Input: part model. Units: mm. Frame: model coordinates. A direction names the side the tool comes from. Coordinates: 2 decimals unless noted, no trailing zeros. Loops run counter-clockwise (first coordinate to the right, second up) from the corner with the lowest first, then second, coordinate; pieces in that order, holes last.
```python
from build123d import *

# Parameters (mm, degrees)
SKETCH_1_R          = 8
SKETCH_1_R_2        = 3
EXTRUDE_1_DEPTH     = 11
SKETCH_2_W          = 1.4
SKETCH_2_H          = 7.329379883
CUT_EXTRUDE_1_DEPTH = 13.5
SKETCH_3_R          = 1
CUT_EXTRUDE_2_DEPTH = 3.5
SKETCH_4_R          = 1.6
EXTRUDE_3_DEPTH     = 2


with BuildPart() as part:
    # 草图1 → 凸台-拉伸1 (new body)
    with BuildSketch(Plane.XY):
        Circle(SKETCH_1_R)
        Circle(SKETCH_1_R_2, mode=Mode.SUBTRACT)
    extrude(amount=EXTRUDE_1_DEPTH)

    # 草图2 → 切除-拉伸1 (cut)
    with BuildSketch(Plane.XY.offset(11)):
        with Locations((0, 5.87801753)):
            Rectangle(SKETCH_2_W, SKETCH_2_H)
    extrude(amount=-CUT_EXTRUDE_1_DEPTH, mode=Mode.SUBTRACT)

    # 草图3 → 切除-拉伸2 (cut)
    with BuildSketch(Plane.XY.offset(11)):
        with Locations((6.5, 0)):
            Circle(SKETCH_3_R)
        with Locations((-6.5, 0)):
            Circle(SKETCH_3_R)
    extrude(amount=-CUT_EXTRUDE_2_DEPTH, mode=Mode.SUBTRACT)

    # 草图4 → 凸台-拉伸3 (add)
    with BuildSketch(Plane.XY.offset(11)):
        with Locations(Location((4.596194078, 4.596194078, 0), (0, 0, 67.691377582))):
            Circle(SKETCH_4_R)
        with Locations(Location((4.596194078, -4.596194078, 0), (0, 0, 292.308622418))):
            Circle(SKETCH_4_R)
        with Locations(Location((-4.596194078, -4.596194078, 0), (0, 0, 202.308622418))):
            Circle(SKETCH_4_R)
        with Locations(Location((-4.596194078, 4.596194078, 0), (0, 0, 157.691377582))):
            Circle(SKETCH_4_R)
    extrude(amount=EXTRUDE_3_DEPTH)


solid = part.part
```
Item 1: Line query: L1, parallel to X at y = 0, z = 5.5; L2, parallel to Y at x = 0, z = 5.5; L3, parallel to Z at x = -5.25, y = -2.75. Output: solid intervals per line, ascending.
Result:
L1: x = -8 to -3, 3 to 8
L2: y = -8 to -3
L3: z = 0 to 11
Item 2: Mould query, pull axis X, two halves, no side actions, for faces 4 (the face through (-0.1, -3.5, 0)), 5 (the face through (0, -8, 5)), 6 (the face through (-0.7, 5, 6)). Classes: +X half, -X half, draft (parallel to the pull), parting line (faces both ways), or undercut.
Result:
face 4: draft
face 5: parting line
face 6: undercut
Item 3: Section query D-D (y = 4.5). Output: boundary loops of the cut face in (x, z), then the cut area to 3 significant figures.
Result:
outline: (-6.61, 0) - (-0.7, 0) - (-0.7, 11) - (-3, 11) - (-3, 13) - (-6.19, 13) - (-6.19, 11) - (-6.61, 11) - close; (0.7, 0) - (6.61, 0) - (6.61, 11) - (6.19, 11) - (6.19, 13) - (3, 13) - (3, 11) - (0.7, 11) - close
area: 143 mm2
Item 4: Reachability of faces 1 (the face through (-3.05, 5.01, 11.99)), 2 (the face through (5, -5, 13)), 3 (the face through (0.7, 5, 6)) from +Z, -Z, +X, -X, +Y, -Y: full face, straight path, thin tool, end or side. Return the list, or none.
Result:
face 1: +Z
face 2: +Z, +X, -X, +Y, -Y
face 3: +Z, -Z, +Y
Item 5: Section query B-B (x = -2.25). Output: boundary loops of the cut face in (y, z), then the cut area to 3 significant figures.
Result:
outline: (-7.68, 0) - (-1.98, 0) - (-1.98, 11) - (-7.68, 11) - close; (1.98, 0) - (7.68, 0) - (7.68, 11) - (1.98, 11) - close
area: 125 mm2
Item 6: Section query C-C (z = 10.5). Output: boundary loops of the cut face in (x, y), then the cut area to 3 significant figures.
Result:
outline: (-0.7, 2.92) - (-0.7, 7.97) arc R8 ccw (long way) to (0.7, 7.97) - (0.7, 2.92) arc R3 cw (long way) to start; hole circle Ø2 at (-6.5, 0); hole circle Ø2 at (6.5, 0)
area: 159 mm2
Item 7: Section query A-A (y = 0). Output: boundary loops of the cut face in (x, z), then the cut area to 3 significant figures.
Result:
outline: (-8, 0) - (-3, 0) - (-3, 11) - (-5.5, 11) - (-5.5, 7.5) - (-7.5, 7.5) - (-7.5, 11) - (-8, 11) - close; (3, 0) - (8, 0) - (8, 11) - (7.5, 11) - (7.5, 7.5) - (5.5, 7.5) - (5.5, 11) - (3, 11) - close
area: 96.0 mm2
Item 8: Contact query for flat-ended pins moving along their axis: P1, Ø1.6, axis at x = -6.5, y = 0, coming from the +Z side; P2, Ø4, axis at y = -2.5, z = 10.5, coming from the +X side; P3, Ø3, axis at y = -5, z = 10, coming from the -X side. Output: stop coordinate, or through.
Result:
P1: stops at z = 7.5
P2: stops at x = 7.98
P3: stops at x = -7.19
